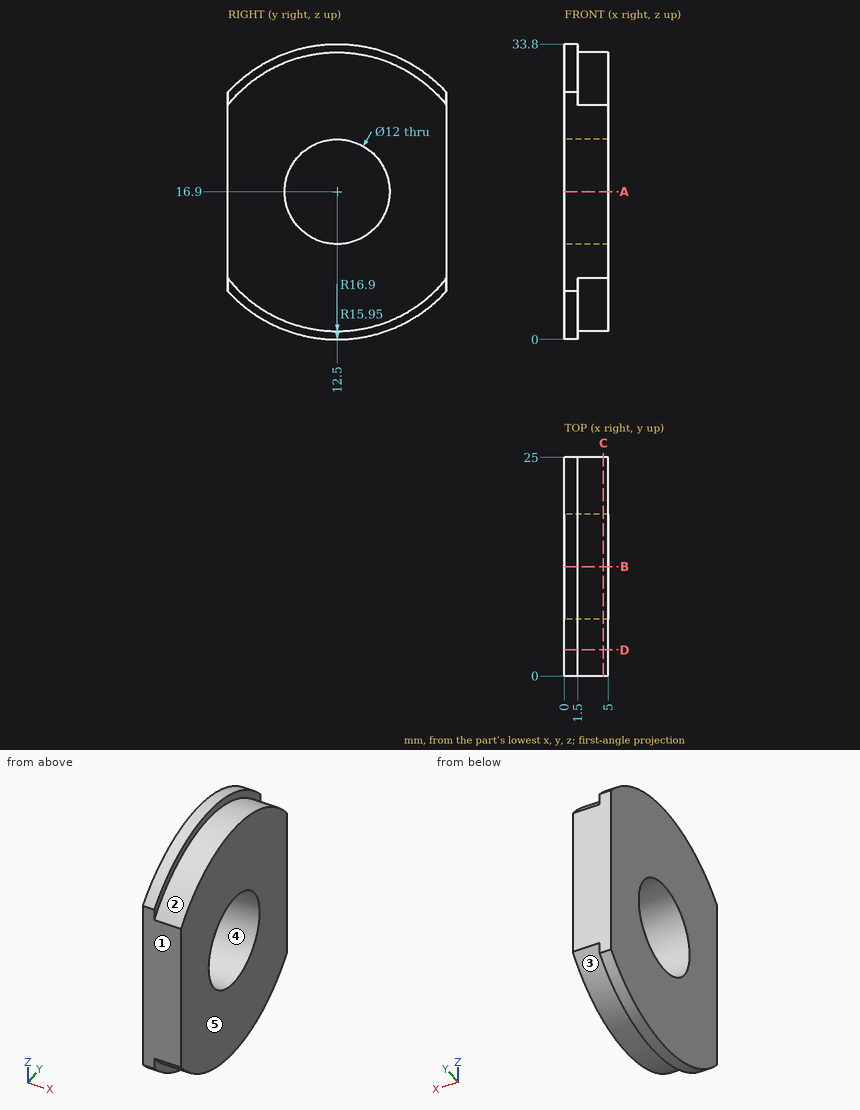
The figure shows three views and two pictorial views of one solid part (mm, origin at its lowest corner). Answer the questions. A direction names the side the tool comes from. Give positions to 0.01 mm unless a question says otherwise; leave off trailing zeros. Loops run counter-clockwise (first coordinate to the right, second up) from the corner with the lowest first, then second, coordinate; pieces in that order, holes last. Notation, with made-up numbers: (55, 68) -> (69, 68) arc R15 ccw to (69, 78) -> close; hole circle Ø2 at (89, -40). An arc over 180 degrees is marked (long way). Put each result on its own line as item: value. Start each with the question number.
Item 1: The part is cut by section A-A (z = 16.9). Give the vertices of the cut face in (x, y).
Item 2: The part is cut by section B-B (y = 12.5). Give the vertices of the cut face in (x, z).
Item 3: Which of the six approach directions +Z, -Z, +X, -X, +Y, -Y give full straight-line access (tool end or side, diameter ignored) to the marked faces 1 and 2?
Item 4: The mould has two halves that part along Y. Classify the marked faces 3, 4 and 5: released by +Y, released by -Y, zero draft, split by the parting line, or undercut.
Item 5: The part is cut by section D-D (y = 3). Give the vertices of the cut face in (x, z), then the cut area to 3 significant figures.
Item 6: The part is cut by section C-C (x = 4.45). Give the vertices of the cut face in (y, z), then the cut area to 3 significant figures.
Item 7: Find the intervals of material crossed by L1, parallel to Z at x = 2, y = 12.5; L2, parallel to Z at x = 2.3, y = 14; L3, parallel to Y at x = 3.95, z = 18, in increasing order. Write a range as [from, to].
Answers below:
1. outline: (0, 0) -> (5, 0) -> (5, 6.5) -> (0, 6.5) -> close; (0, 18.5) -> (5, 18.5) -> (5, 25) -> (0, 25) -> close
2. outline: (0, 0) -> (1.5, 0) -> (1.5, 0.95) -> (5, 0.95) -> (5, 10.9) -> (0, 10.9) -> close; (0, 22.9) -> (5, 22.9) -> (5, 32.85) -> (1.5, 32.85) -> (1.5, 33.8) -> (0, 33.8) -> close
3. face 1: +Z, -Z, +X, -X, -Y
3. face 2: +Z, +X
4. face 3: split by the parting line
4. face 4: undercut
4. face 5: zero draft
5. outline: (0, 2.92) -> (1.5, 2.92) -> (1.5, 4.09) -> (5, 4.09) -> (5, 29.71) -> (1.5, 29.71) -> (1.5, 30.88) -> (0, 30.88) -> close
5. area: 132 mm2
6. outline: (0, 6.99) arc R15.95 ccw to (25, 6.99) -> (25, 26.81) arc R15.95 ccw to (0, 26.81) -> close; hole circle Ø12 at (12.5, 16.9)
6. area: 593 mm2
7. L1: [0.95, 10.9], [22.9, 32.85]
7. L2: [1.02, 11.09], [22.71, 32.78]
7. L3: [0, 6.6], [18.4, 25]
